```python
from build123d import *

# Parameters (mm, degrees)
SKETCH_1_W      = 21
SKETCH_1_H      = 42.43
SKETCH_1_R      = 2.6
EXTRUDE_1_DEPTH = 3
FILLET_1_R      = 10


with BuildPart() as part:
    # 草图1 → 凸台-拉伸1 (new body)
    # profile 1 of 3: a face of its own
    with BuildSketch(Plane(origin=(0, 0, 0), x_dir=(1, 0, 0), z_dir=(0, 1, 0))):
        with Locations((-139.5, 0)):
            Rectangle(SKETCH_1_W, SKETCH_1_H)
        with Locations(Location((-132.3, 0, 0), (0, 0, 270))):
            Circle(SKETCH_1_R, mode=Mode.SUBTRACT)
    # profile 2 of 3: a face of its own
    with BuildSketch(Plane(origin=(0, 0, 0), x_dir=(1, 0, 0), z_dir=(0, 1, 0))):
        with BuildLine():
            Line((129, 21.215), (-129, 21.215))
            Line((-129, 21.215), (-129, -21.215))
            Line((-129, -21.215), (129, -21.215))
            Line((129, -21.215), (129, -2.4))
            ThreePointArc((129, -2.4), (127.4, 0), (129, 2.4))
            Line((129, 2.4), (129, 21.215))
        make_face()
    # profile 3 of 3: a face of its own
    with BuildSketch(Plane(origin=(0, 0, 0), x_dir=(1, 0, 0), z_dir=(0, 1, 0))):
        with BuildLine():
            Line((150, 21.215), (129, 21.215))
            Line((129, 21.215), (129, 2.4))
            ThreePointArc((129, 2.4), (131.44222051, 2.163330765), (132.6, 0))
            ThreePointArc((132.6, 0), (131.44222051, -2.163330765), (129, -2.4))
            Line((129, -2.4), (129, -21.215))
            Line((129, -21.215), (150, -21.215))
            Line((150, -21.215), (150, 21.215))
        make_face()
    extrude(amount=EXTRUDE_1_DEPTH)

    # 圆角1
    # the kernel refuses this fillet: 10 mm, written as the material it takes off along each edge
    with BuildSketch(Plane(origin=(150, 3, 39.068571071), x_dir=(-1, 0, 0), z_dir=(0, 0, -1)), Plane(origin=(-150, 3, -39.068571071), x_dir=(1, 0, 0), z_dir=(0, 0, 1))) as fillet_1_piece_1:
        with BuildLine():
            CenterArc((7.141428429, -10), FILLET_1_R, 90, 45.572995999)
            Line((0, -3), (-0.142828569, -2.86))
            ThreePointArc((-0.142828569, -2.86), (-0.2, -1.5), (-0.2, 0))
            Line((-0.2, 0), (0, 0.2))
            Line((0, 0.2), (7.141428429, 0.2))
            Line((7.141428429, 0.2), (7.141428429, 0))
        make_face()
    extrude(amount=78.137142143, mode=Mode.SUBTRACT)
    with BuildSketch(Plane(origin=(-167.853571071, 3, 21.215), x_dir=(0, 0, -1), z_dir=(1, 0, 0))) as fillet_1_piece_2:
        with BuildLine():
            CenterArc((7.141428429, -10), FILLET_1_R, 90, 45.572995999)
            Line((0, -3), (-0.142828569, -2.86))
            ThreePointArc((-0.142828569, -2.86), (-0.2, -1.5), (-0.2, 0))
            Line((-0.2, 0), (0, 0.2))
            Line((0, 0.2), (7.141428429, 0.2))
            Line((7.141428429, 0.2), (7.141428429, 0))
        make_face()
    extrude(amount=335.707142143, mode=Mode.SUBTRACT)
    with BuildSketch(Plane(origin=(-167.853571071, 3, -21.215), x_dir=(0, -1, 0), z_dir=(1, 0, 0))) as fillet_1_piece_3:
        with BuildLine():
            CenterArc((10, -7.141428429), FILLET_1_R, 134.427004001, 45.572995999)
            Line((0, -7.141428429), (-0.2, -7.141428429))
            Line((-0.2, -7.141428429), (-0.2, 0))
            Line((-0.2, 0), (0, 0.2))
            ThreePointArc((0, 0.2), (1.5, 0.2), (2.86, 0.142828569))
            Line((2.86, 0.142828569), (3, 0))
        make_face()
    extrude(amount=335.707142143, mode=Mode.SUBTRACT)


solid = part.part
```
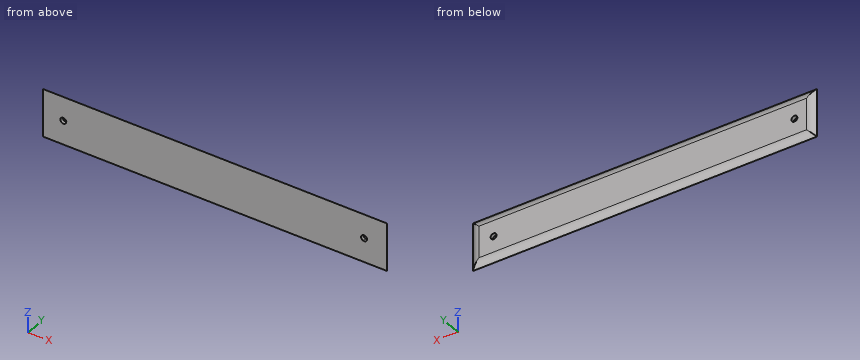
For this review, take the finished solid that the model builds, in its own axes (mm). Give positions to 0.01 mm unless a question says otherwise; leave off trailing zeros. Write each loop counter-clockwise with the first axis right and the second up, starting at its lowest first coordinate (ties: lowest second). Pieces come first, ordered by that corner, then holes. Notation, with made-up numbers: M 70.25,63.25 L 83.25,63.25 A16 ccw 83.25,80.25 Z; hole C 3,75.25 d4. An arc over 180 degrees is marked long. One line per item, written item: value.
1) Take a section at A-A, the plane x = -132.3. Write out the cut boundary in (y, z) (3 decimals).
Results are:
outline: M 0,-21.215 A10 ccw 3,-14.074 L 3,-2.6 L 0,-2.6 Z; M 0,2.6 L 3,2.6 L 3,14.074 A10 ccw 0,21.215 Z
2) For line 1 (X direction, y = 1.55, z = 0); line 2 (X direction, y = 0.5, z = 1.5); line 3 (Z direction, x = -132.3, y = 0.75), list the stretches that pass through material, from the lowest coordinate up. Write a range as from..to.
Results are:
line 1: x = -148.04..-134.9, -129.7..127.4, 132.6..148.04
line 2: x = -149.47..-134.42, -130.18..127.88, 132.12..149.47
line 3: z = -20.39..-2.6, 2.6..20.39
3) For P1, Ø1, axis at x = 28, y = 1, coming from the -Z side; P2, Ø1.5, axis at y = 1, z = -15.5, coming from the -X side, all flat-tipped, find the tip position at first contact; note any pin that passes through.
Results are:
P1: stops at z = -20.69
P2: stops at x = -149.75
4) Take a section at C-C, the plane x = -58. Write out the cut boundary in (y, z) (3 decimals), then the cut area to 3 significant figures.
Results are:
outline: M 0,-21.215 A10 ccw 3,-14.074 L 3,14.074 A10 ccw 0,21.215 Z
area: 114 mm²
5) Take a section at B-B, the plane y = 2.55. Write out the cut boundary in (x, z).
Results are:
outline: M -145.82,-17.04 L 145.82,-17.04 L 145.82,17.04 L -145.82,17.04 Z; hole C -132.3,0 d5.2; hole C 130,0 d5.2
